Here's how the part is built. I have some questions about the finished solid (model axes, mm). Face numbers are marked on the shaded views. A direction names the side the tool comes from. Coordinates: 2 decimals unless noted, no trailing zeros. Loops run counter-clockwise (first coordinate to the right, second up) from the corner with the lowest first, then second, coordinate; pieces in that order, holes last. Notation, with made-up numbers: M 32.5,41.25 L 45.5,41.25 A21 cw 45.5,67.25 Z; hole C -8,70 d8. An arc over 180 degrees is marked long. Use CSV: the item, a comma, the result in double quotes. Start each with the question number.
Q1. If we section it at B-B (x = -27): Please give me the cut outline in (y, z).
Q2. For pin 1 Ø8 at (x, z) = (27, -20.5) entering from -Y; pin 2 Ø6 at (x, z) = (-15.5, -24) entering from -Y; pin 3 Ø10 at (x, y) = (-1, -38) entering from +Z, each with a flat end and sliding along its axis, tell me the tip position at first contact or that it passes through.
Q3. If we section it at C-C (x = 0): Please give me the cut outline in (y, z), and give its area (3 significant figures).
Q4. If we mould it in two halves opening along Y, with no side actions, what happens to the marked faces 4, 5, 6 and 7? For each: +Y half, -Y half, draft (parallel to the pull), parting line (faces both ways), or undercut.
Q5. Which directions (+Z, -Z, +X, -X, +Y, -Y) give clear straight access to the entire face, cutting with the end or side of a thin tool? Please do the marked faces 1, 2 and 3.
Q6. If we section it at A-A (y = -15): Please give me the cut outline in (x, z).
Q7. Please list where these lines run through material, in increasing order: probe 1 along X at (y, z) = (-33, -16.5); probe 2 along Y at (x, z) = (54.5, -25); probe 3 along X at (y, z) = (-45, -6.5). Write a range as [from, to].
Q8. If we section it at D-D (y = -54.5): Please give me the cut outline in (x, z).
from build123d import *

# Parameters (mm, degrees)
SKETCH2_W              = 115
SKETCH2_H              = 5
BOSS_EXTRUDE1_DEPTH    = 50
SKETCH3_W              = 5
SKETCH3_H              = 50
BOSS_EXTRUDE2_DEPTH    = 100
CUT_EXTRUDE1_DEPTH     = 162.960643367
SKETCH5_R              = 2.5
CUT_EXTRUDE2_DEPTH     = 162.960643367
CUT_EXTRUDE3_START     = -5
CUT_EXTRUDE3_OUTLINE_R = 7.5
CUT_EXTRUDE3_DEPTH     = 5
SKETCH7_W              = 2
SKETCH7_H              = 20
BOSS_EXTRUDE3_DEPTH    = 40
SKETCH8_W              = 20
SKETCH8_H              = 2
BOSS_EXTRUDE4_DEPTH    = 52
BOSS_EXTRUDE6_REACH    = 100.236
SKETCH9_W              = 2
SKETCH9_H              = 20


# Read off the part's stored shape, not the designer's step: Cut-Extrude3
with BuildPart() as part:
    # Sketch2 → Boss-Extrude1 (new body)
    with BuildSketch(Plane.XY):
        Rectangle(SKETCH2_W, SKETCH2_H)
    extrude(amount=-BOSS_EXTRUDE1_DEPTH)

    # Sketch3 → Boss-Extrude2 (add)
    with BuildSketch(Plane.XZ.offset(2.5)):
        with Locations((-55, -25)):
            Rectangle(SKETCH3_W, SKETCH3_H)
        with Locations((55, -25)):
            Rectangle(SKETCH3_W, SKETCH3_H)
    extrude(amount=BOSS_EXTRUDE2_DEPTH)

    # Sketch4 → Cut-Extrude1 (cut, through all)
    with BuildSketch(Plane.ZY.offset(57.5)):
        with BuildLine():
            Line((0, -102.5), (0, -77.5))
            ThreePointArc((0, -77.5), (-7.32233047, -95.17766953), (-25, -102.5))
            Line((-25, -102.5), (0, -102.5))
        make_face()
        with BuildLine():
            ThreePointArc((-25, -102.5), (-42.67766953, -95.17766953), (-50, -77.5))
            Line((-50, -77.5), (-50, -102.5))
            Line((-50, -102.5), (-25, -102.5))
        make_face()
    extrude(amount=-CUT_EXTRUDE1_DEPTH, mode=Mode.SUBTRACT)

    # Sketch5 → Cut-Extrude2 (cut, through all)
    with BuildSketch(Plane.ZY.offset(57.5)):
        with Locations((-25, -77.5)):
            Circle(SKETCH5_R)
    extrude(amount=-CUT_EXTRUDE2_DEPTH, mode=Mode.SUBTRACT)

    # Cut-Extrude3 outline → Cut-Extrude3 (cut)
    with BuildSketch(Plane.XZ.offset(2.5).offset(CUT_EXTRUDE3_START)):
        with Locations((0, -25)):
            Circle(CUT_EXTRUDE3_OUTLINE_R)
    extrude(amount=CUT_EXTRUDE3_DEPTH, mode=Mode.SUBTRACT)

    # Sketch7 → Boss-Extrude3 (add)
    with BuildSketch(Plane.XZ.offset(2.5)):
        with Locations((21, -25)):
            Rectangle(SKETCH7_W, SKETCH7_H)
    extrude(amount=BOSS_EXTRUDE3_DEPTH)

    # Sketch8 → Boss-Extrude4 (add)
    with BuildSketch(Plane.ZY.offset(-20)):
        with Locations((-25, -41.5)):
            Rectangle(SKETCH8_W, SKETCH8_H)
    extrude(amount=BOSS_EXTRUDE4_DEPTH)

    # Sketch9 → Boss-Extrude6 (add, up to next)
    with BuildSketch(Plane(origin=(0, -40.5, 0), x_dir=(1, 0, 0), z_dir=(0, 1, 0)), mode=Mode.PRIVATE) as boss_extrude6_sk1:
        with Locations((-31, 25)):
            Rectangle(SKETCH9_W, SKETCH9_H)
    boss_extrude6_tool1 = extrude(boss_extrude6_sk1.sketch, amount=BOSS_EXTRUDE6_REACH, mode=Mode.PRIVATE) - part.part
    add(boss_extrude6_tool1.solids().sort_by_distance((-31, -40.5, -25))[0])


solid = part.part
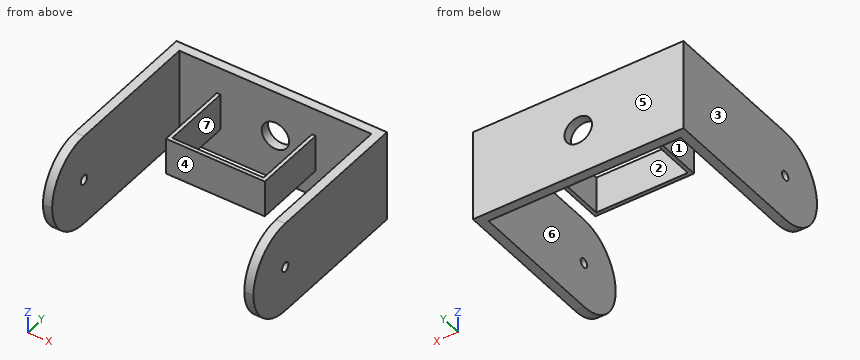
Results below:
1,outline,"M -42.5,-35 L -40.5,-35 L -40.5,-15 L -42.5,-15 Z; M -2.5,-50 L 2.5,-50 L 2.5,0 L -2.5,0 Z"
2,pin 1,"y = -2.5"
2,pin 2,"y = -42.5"
2,pin 3,"z = -15"
3,outline,"M -42.5,-35 L -40.5,-35 L -40.5,-15 L -42.5,-15 Z; M -2.5,-50 L 2.5,-50 L 2.5,-32.5 L -2.5,-32.5 Z; M -2.5,-17.5 L 2.5,-17.5 L 2.5,0 L -2.5,0 Z"
3,area,"215 mm^2"
4,face 4,"-Y half"
4,face 5,"+Y half"
4,face 6,"draft"
4,face 7,"undercut"
5,face 1,"+Z, -Z, -Y"
5,face 2,"+Z, -Z"
5,face 3,"+Z, -Z, -X, +Y, -Y"
6,outline,"M -57.5,-50 L -52.5,-50 L -52.5,0 L -57.5,0 Z; M -32,-35 L -30,-35 L -30,-15 L -32,-15 Z; M 20,-35 L 22,-35 L 22,-15 L 20,-15 Z; M 52.5,-50 L 57.5,-50 L 57.5,0 L 52.5,0 Z"
7,probe 1,"[-57.5, -52.5], [-32, -30], [20, 22], [52.5, 57.5]"
7,probe 2,"[-102.5, -80], [-75, 2.5]"
7,probe 3,"[-57.5, -52.5], [52.5, 57.5]"
8,outline,"M -57.5,-50 L -52.5,-50 L -52.5,0 L -57.5,0 Z; M 52.5,-50 L 57.5,-50 L 57.5,0 L 52.5,0 Z"
